```python
from build123d import *

# Parameters (mm, degrees)
F0_R      = 50
F1_DEPTH  = 25
F3_D      = 10
F5_DEPTH  = 5
F7_DEPTH  = 10
F9_DEPTH  = 5
F11_DEPTH = 5
F13_D     = 5
F15_DEPTH = 5
F17_DEPTH = 5
F19_DEPTH = 5
F21_D     = 5


with BuildPart() as f1:
    # F0 (on Front) → F1 (new body)
    with BuildSketch(Plane.XZ):
        Circle(F0_R)
    extrude(amount=F1_DEPTH)

    # F3 (through all)
    with Locations(Plane.XZ.offset(25)):
        with Locations((0, 0)):
            Hole(F3_D / 2)

    # F4 (on face) → F5 (join)
    with BuildSketch(Plane.XZ.offset(25)):
        Polygon((-1, 5), (0, 5), (0, 12.4759720638), (12.0539031955, 12.4759720638), (12.0539031955, 0), (12.0539031955, -10.0090857595), (0, -10.0090857595), (-11.5974724069, -10.0090857595), (-11.5974724069, 0), (-11.5974724069, 12.4759720638), (-11.5974724069, 21.0507828742), (22.3206661865, 21.0507828742), (22.3206661865, 22.0507828742), (-11.5974724069, 22.0507828742), (-12.5974724069, 22.0507828742), (-12.5974724069, 5.5559086613), (-12.5974724069, -11.0117533952), (13.2704021633, -11.0090857595), (13.2704021633, -10.0090857595), (13.2704021633, 12.4759720638), (13.2704021633, 13.4759720638), (0, 13.4759720638), (-1, 13.4759720638), (-1, 12.4759720638), align=None)
        Polygon((-16.5974722952, 12.4759720638), (-16.5974722952, 26.0507827625), (22.3206661865, 26.0507827625), (22.3206661865, 27.0507827625), (-16.5974722952, 27.0507827625), (-17.5974722952, 27.0507827625), (-17.5974722952, 26.1644367129), (-17.5974722952, -14.8946940899), (-17.5974722952, -15.0090856478), (-17.5974722952, -16.0090856478), (18.0539030838, -16.0090856478), (18.0539030838, -15.0090856478), (18.0539030838, 18.475971811), (17.0539030838, 18.475971811), (-4.9999998818, 18.4759719521), (-4.9999998882, 17.4759719521), (-4.9999998882, 5), (-3.9999998882, 5), (-3.9999998882, 17.4759719521), (17.0539030838, 17.4759719521), (17.0539030838, 0), (17.0539030838, -15.0090856478), (-0.0038306937, -15.0090856478), (-16.5974722952, -15.0090856478), (-16.5974722952, 0), align=None)
    extrude(amount=F5_DEPTH)

    # F6 (on face) → F7 (join)
    with BuildSketch(Plane.XZ.offset(25)):
        with BuildLine():
            Line((-3.9999998882, 5), (-4.9999998882, 5))
            Line((-4.9999998882, 5), (-4.9999999831, 0.7558615648))
            Line((-4.9999999831, 0.7558615648), (-4.9053492841, 0.9682708303))
            ThreePointArc((-4.9053492841, 0.9682708303), (-4.5670879099, 2.0351186755), (-3.9999998882, 3.000000149))
            Line((-3.9999998882, 3.000000149), (-3.9999998882, 5))
        make_face()
    extrude(amount=F7_DEPTH)

    # F8 (on face) → F9 (join)
    with BuildSketch(Plane.XZ.offset(25)):
        Polygon((25.6022717804, 27.0507827625), (22.3206661865, 27.0507827625), (22.3206661865, 26.0507827625), (25.6022717804, 26.0507827625), (27.1489042789, 26.0507827625), (28.8951024413, 26.0507827625), (32.8879207373, 26.0507827625), (32.8879207373, 18.475971811), (32.8879207373, 9.354759939), (32.8879207373, 5.5606500246), (32.8879207373, 0), (32.8879207373, -5.7792388834), (32.8879207373, -17.5537280738), (32.8879207373, -21.467147395), (32.8879207373, -23.2733413577), (34.0968593955, -23.2733413577), (34.0968593955, -16.0090856478), (34.0968593955, 0), (34.0968593955, 6.9746486843), (34.0968593955, 11.9728827849), (34.0968593955, 18.475971811), (34.0968593955, 27.0507827625), (32.8879207373, 27.0507827625), (28.4710265696, 27.0507827625), align=None)
    extrude(amount=F9_DEPTH)

    # F10 (on face) → F11 (join)
    with BuildSketch(Plane.XZ.offset(25)):
        Polygon((34.0968593955, -23.2733413577), (32.8879207373, -23.2733413577), (0, -23.2733413577), (0, -26.040263474), (34.0968593955, -26.040263474), align=None)
    extrude(amount=F11_DEPTH)

    # F13 (through all)
    with Locations(Plane.XZ.offset(25)):
        with Locations((25.2206400037, -16.9608648866), (28.3664222807, 16.152607277)):
            Hole(F13_D / 2)

    # F14 (on face) → F15 (join)
    with BuildSketch(Plane.XZ.offset(25)):
        Polygon((-28.4231826663, 31.7307532181), (-38.6414194901, 31.7307532181), (-38.6414194901, -31.7307532181), (-28.4231826663, -31.7307532181), (-28.4231826663, -31.0340896249), align=None)
    extrude(amount=F15_DEPTH)

    # F16 (on face) → F17 (join)
    with BuildSketch(Plane.XZ.offset(25)):
        Polygon((-19.8692139238, -28.657739982), (-28.4231826663, -13.8425510377), (-28.4231826663, -28.657739982), align=None)
        Polygon((-19.8692139238, -13.8425510377), (-28.4231826663, 0), (-28.4231826663, -13.8425510377), align=None)
        Polygon((-19.8692139238, 0), (-28.4231826663, 14.5734706894), (-28.4231826663, 0), align=None)
        Polygon((-19.8692139238, 14.5734706894), (-28.4231826663, 31.7307532181), (-28.4231826663, 14.5734706894), align=None)
    extrude(amount=F17_DEPTH)

    # F18 (on face) → F19 (join)
    with BuildSketch(Plane.XZ.offset(25)):
        Polygon((-23.9576643267, -30.233348331), (-27.21523121, -33.645581454), (-13.0854109302, -47.1349395812), (-8.995237881, -44.5175730967), align=None)
        Polygon((-8.995237881, -44.5175730967), (-13.0854109302, -47.1349395812), (-5.403298419, -47.1349395812), (5.4181421023, -31.7307532181), (0, -28.657739982), align=None)
    extrude(amount=F19_DEPTH)

    # F21 (through all)
    with Locations(Plane.XZ.offset(25)):
        with Locations((14.6169317886, -33.61049667)):
            Hole(F21_D / 2)


solid = f1.part
```
Source: CAD feature listing. Evaluate the final solid. Frame: model axes, mm. A direction names the side the tool comes from. Give positions to 0.01 mm unless a question says otherwise; leave off trailing zeros. Loops run counter-clockwise (first coordinate to the right, second up) from the corner with the lowest first, then second, coordinate; pieces in that order, holes last. Notation, with made-up numbers: (62, 50) - (100, 50) arc R14 ccw to (100, 72) - close; hole circle Ø5 at (4, 80). An arc over 180 degrees is marked (long way). Use CSV: the item, a comma, the result in double quotes.
1) Pin query (flat end, axial travel): P1, Ø6, axis at x = 25.22, z = -16.96, coming from the -Y side; P2, Ø2, axis at x = 38, y = -12, coming from the -Z side; P3, Ø12.5, axis at x = -44.5, z = 14.5, coming from the -Y side; P4, Ø4, axis at x = 28.37, z = 16.15, coming from the +Y side. Return the tip coordinate at first contact, or that it passes through.
Worked out:
P1,"stops at y = -25"
P2,"stops at z = -33.63"
P3,"stops at y = -30"
P4,"passes through"
2) Set-up query: faces 4 (the flat face through (-1, 0, -10)), 5 (the flat face through (-38.641, -27, 0)), 6 (the flat face through (2.747, -27.465, -30.216)), 7 (the flat face through (12.054, -27, 1)). Return all of +Z, -Z, +X, -X, +Y, -Y with unobstructed straight access to the full face (end or side cutting, diameter ignored); none if empty.
Worked out:
face 4,"+Z, -Z, +X, -X, +Y"
face 5,"+Z, -Z, -X, -Y"
face 6,"+X, -Y"
face 7,"-Y"
3) Mould query, pull axis X, two halves, no side actions, for faces 1 (the flat face through (-20.249, -27.465, -40.296)), 2 (the flat face through (-9, -27, -47.135)), 3 (the flat face through (-24.086, -27.465, -7.018)). Classes: +X half, -X half, draft (parallel to the pull), parting line (faces both ways), or undercut.
Worked out:
face 1,"-X half"
face 2,"draft"
face 3,"undercut"
4) Cut plane A-A (y = -5). Output: boundary loops of the cut face in (x, z), and give its area (3 significant figures).
Worked out:
outline,"circle Ø100 at (0, 0); hole circle Ø10 at (0, 0); hole circle Ø5 at (14.62, -33.61); hole circle Ø5 at (25.22, -16.96); hole circle Ø5 at (28.37, 16.15)"
area,"7,720 mm^2"
5) Cut plane B-B (z = -39). Output: boundary loops of the cut face in (x, y), and give its area (3 significant figures).
Worked out:
outline,"(-31.29, -25) - (-21.61, -25) - (-21.61, -30) - (-14.77, -30) - (-14.77, -25) - (-5.87, -25) - (-5.87, -30) - (0.31, -30) - (0.31, -25) - (31.29, -25) - (31.29, 0) - (-31.29, 0) - close"
area,"1,630 mm^2"
6) Line query: line 1 (Y direction, x = -8.5, z = 14); line 2 (Z direction, x = 0, y = -14); line 3 (Y direction, x = -17, z = 18). Output: solid intervals per line, ascending.
Worked out:
line 1,"y = -25 to 0"
line 2,"z = -50 to -5, 5 to 50"
line 3,"y = -30 to 0"
7) Cut plane C-C (x = 37.5). Output: boundary loops of the cut face in (y, z).
Worked out:
outline,"(-25, -33.07) - (0, -33.07) - (0, 33.07) - (-25, 33.07) - close"
